Geometry: final body of the model. Coordinates: model frame, mm. Face numbers are marked on the shaded views. A direction names the side the tool comes from. Coordinates: 2 decimals unless noted, no trailing zeros. Order: outer loops, then holes, each group sorted by start corner. A loop starts at its lowest first (then second) coordinate and runs counter-clockwise, first axis right, second up. Notation, with made-up numbers: (-30.5, 5) - (28.5, 5) arc R34 ccw to (28.5, 35) - close; hole circle Ø11 at (41.25, 81). An arc over 180 degrees is marked (long way). Use a Markdown table: item, result. Add a question column.
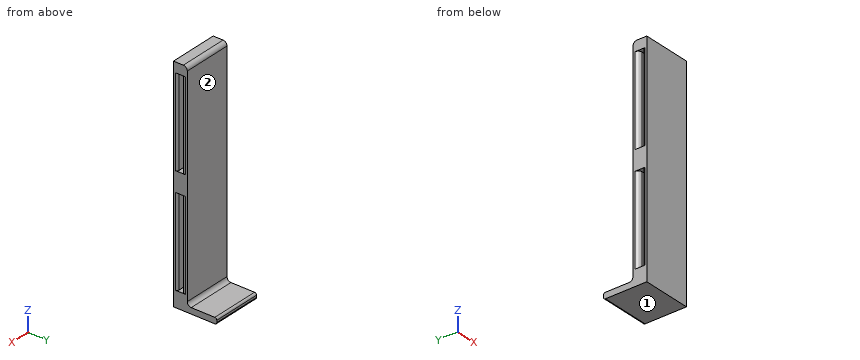
```python
from build123d import *

# Parameters (mm, degrees)
F0_W     = 2
F0_H     = 45
F1_DEPTH = 25
F2_R     = 2
F4_R     = 1


# Not quite as in the source:
# - two fillets or chamfers of one size are made in one step


with BuildPart() as f1:
    # F0 (on Right) → F1 (new body)
    with BuildSketch(Plane.YZ):
        with BuildLine():
            Line((7, 113), (0, 113))
            Line((0, 113), (0, 0))
            Line((0, 0), (21, 0))
            ThreePointArc((21, 0), (21.7071067812, 0.2928932188), (22, 1))
            Line((22, 1), (22, 2))
            ThreePointArc((22, 2), (21.7071067812, 2.7071067812), (21, 3))
            Line((21, 3), (7, 3))
            Line((7, 3), (7, 113))
        make_face()
        with Locations((3, 30.5)):
            Rectangle(F0_W, F0_H, mode=Mode.SUBTRACT)
        with Locations((3, 85.5)):
            Rectangle(F0_W, F0_H, mode=Mode.SUBTRACT)
    extrude(amount=F1_DEPTH)

    # F2 (call 1 of 6: OpenCascade refuses the feature's edges together)
    f2_edges = [f1.edges().sort_by_distance(p)[0] for p in [
        (12.5, 7, 3),
    ]]
    fillet(f2_edges, radius=F2_R)

    # F2#2 (call 2 of 6)
    f2_2_edges = [f1.edges().sort_by_distance(p)[0] for p in [
        (12.5, 7, 113),
    ]]
    fillet(f2_2_edges, radius=F2_R)

    # F2#3 (call 3 of 6)
    f2_3_edges = [f1.edges().sort_by_distance(p)[0] for p in [
        (0, 4, 30.5),
    ]]
    fillet(f2_3_edges, radius=F2_R)

    # F2#4 (call 4 of 6)
    f2_4_edges = [f1.edges().sort_by_distance(p)[0] for p in [
        (25, 4, 30.5),
    ]]
    fillet(f2_4_edges, radius=F2_R)

    # F2#5 (call 5 of 6)
    f2_5_edges = [f1.edges().sort_by_distance(p)[0] for p in [
        (0, 4, 85.5),
    ]]
    fillet(f2_5_edges, radius=F2_R)

    # F2#6 (call 6 of 6)
    f2_6_edges = [f1.edges().sort_by_distance(p)[0] for p in [
        (25, 4, 85.5),
    ]]
    fillet(f2_6_edges, radius=F2_R)

    # F4
    f4_edges = [f1.edges().sort_by_distance(p)[0] for p in [
        (25, 2, 30.5),
        (25, 2, 85.5),
        (0, 2, 85.5),
        (0, 2, 30.5),
    ]]
    fillet(f4_edges, radius=F4_R)


solid = f1.part
```
1) Section query C-C (y = 13). Return the cut outline in (x, z), and give its area (3 significant figures).
2) Access query for the marked faces 1 and 2. Directions: +Z, -Z, +X, -X, +Y, -Y. A direction counts if a zero-diameter tool reaches every point of the face in a straight line with its end or side. Return the directions, or none.
3) First-contact query: pin 1 (1.5 mm diameter, centred on x = 5, z = 47, fed in from +Y); pin 2 (6 mm diameter, centred on x = 17.5, y = 14.5, fed in from +Z). Flat tips, straight axial feed; report the tip coordinate or a pass-through.
4) Section query A-A (z = 79). Return the cut outline in (x, y), and give its area (3 significant figures).
5) Line query: line 1 (Z direction, x = 18.5, y = 3.5); line 2 (Y direction, x = 22.5, z = 25.5); line 3 (Z direction, x = 21.25, y = 12.75). Output: solid intervals per line, ascending. Write a range as from..to.
6) Section query D-D (z = 55). Return the cut outline in (x, y).
7) Section query B-B (x = 12.25). Return the cut outline in (y, z).
From the geometry:
| question | item | result |
|---|---|---|
| 1 | outline | (0, 0) - (25, 0) - (25, 3) - (0, 3) - close |
| 1 | area | 75.0 mm^2 |
| 2 | face 1 | -Z, +X, -X, +Y, -Y |
| 2 | face 2 | +Z, +X, -X, +Y |
| 3 | pin 1 | stops at y = 7 |
| 3 | pin 2 | stops at z = 3 |
| 4 | outline | (0, 0) - (25, 0) - (25, 1) arc R1 ccw to (24, 2) - (1, 2) arc R1 ccw to (0, 1) - close; (0, 6) arc R2 ccw to (2, 4) - (23, 4) arc R2 ccw to (25, 6) - (25, 7) - (0, 7) - close |
| 4 | area | 123 mm^2 |
| 5 | line 1 | z = 0..8, 53..63, 108..113 |
| 5 | line 2 | y = 0..2, 4..7 |
| 5 | line 3 | z = 0..3 |
| 6 | outline | (0, 0) - (25, 0) - (25, 7) - (0, 7) - close |
| 7 | outline | (0, 0) - (21, 0) arc R1 ccw to (22, 1) - (22, 2) arc R1 ccw to (21, 3) - (9, 3) arc R2 cw to (7, 5) - (7, 111) arc R2 ccw to (5, 113) - (0, 113) - close; hole (2, 8) - (4, 8) - (4, 53) - (2, 53) - close; hole (2, 63) - (4, 63) - (4, 108) - (2, 108) - close |
